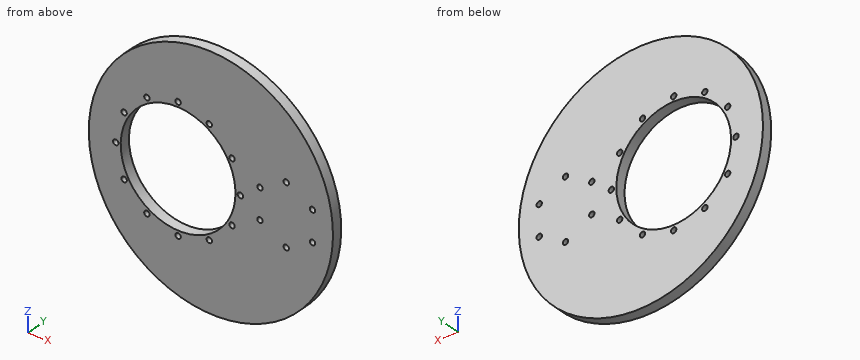
from build123d import *

# Parameters (mm, degrees)
SKETCH1_R                       = 74.45
SKETCH1_R_2                     = 35
BOSS_EXTRUDE1_DEPTH             = 6.35
M4X0_7_TAPPED_HOLE1_D           = 3.3
M4X0_7_TAPPED_HOLE1_ON_FACE_2_D = 3.3


with BuildPart() as part:
    # Sketch1 → Boss-Extrude1 (new body)
    with BuildSketch(Plane(origin=(0, 0, 0), x_dir=(1, 0, 0), z_dir=(0, 1, 0))):
        with Locations(Location((20, 0, 0), (0, 0, 270))):
            Circle(SKETCH1_R)
        with Locations(Location((0, 0, 0), (0, 0, 270))):
            Circle(SKETCH1_R_2, mode=Mode.SUBTRACT)
    extrude(amount=BOSS_EXTRUDE1_DEPTH)

    # M4x0.7 Tapped Hole1 (through all)
    with Locations(Plane(origin=(0, 0, -38), x_dir=(0, 0, -1), z_dir=(0, -1, 0))):
        with Locations((0, 0), (-5.091034656, -19), (-19, -32.908965344), (-38, -38), (-57, -32.908965344), (-70.908965344, -19), (-76, 0), (-70.908965344, 19), (-57, 32.908965344), (-38, 38), (-5.091034656, 19), (-19, 32.908965344)):
            Hole(M4X0_7_TAPPED_HOLE1_D / 2)

    # M4x0.7 Tapped Hole1 on face 2 (through all)
    with Locations(Plane(origin=(65.95, 6.35, -18.5), x_dir=(0, 0, 1), z_dir=(0, 1, 0))):
        with Locations((0, 0), (9.25, 16.02146997), (27.75, 16.02146997), (37, 0), (27.75, -16.02146997), (9.25, -16.02146997)):
            Hole(M4X0_7_TAPPED_HOLE1_ON_FACE_2_D / 2)


solid = part.part
Work out the finished part from the listing and answer in its coordinate system (mm). Round coordinates to 2 decimals unless told otherwise and drop trailing zeros. Loops run counter-clockwise (first coordinate to the right, second up) from the corner with the lowest first, then second, coordinate; pieces in that order, holes last. Notation, with made-up numbers: (73.25, 36.25) - (98.25, 36.25) arc R18 cw to (98.25, 68.25) - close; hole circle Ø8 at (8.5, 19.25). An arc over 180 degrees is marked (long way). Use one line per item in the form item = value. Start each with the question number.
(1) Find section A-A on x = -12. Determine the outline of the cut face in (y, z).
(2) Find section B-B on y = 4.25. Give the number of separate pieces and of enclosed holes in the cut face, and give its area (3 significant figures).
(3) Find section D-D on x = 69.5. Determine the outline of the cut face in (y, z), and give its area (3 significant figures).
(4) Flat-ended cylindrical pins translate along their axes: P1, Ø1.5, axis at x = 43.5, y = 1, coming from the -Z side; P2, Ø1.5, axis at y = 4, z = -50, coming from the -X side; P3, Ø3, axis at x = 25.5, y = 2, coming from the +Z side. Find the tip coordinate at first contact, or state that the pin passes through.
(5) Find section C-C on z = 42. Determine the outline of the cut face in (x, y).
(6) Consider line 1 (X direction, y = 3, z = 0); line 2 (Z direction, x = 51, y = 4); line 3 (Z direction, x = 67, y = 5). Determine where each line is inside the solid, lowest interval first.
Answer list:
q1.outline = (0, -67.22) - (6.35, -67.22) - (6.35, -32.88) - (0, -32.88) - close; (0, 32.88) - (6.35, 32.88) - (6.35, 67.22) - (0, 67.22) - close
q2.separate_pieces = 1
q2.enclosed_holes = 19
q2.area = 13,400 mm^2
q3.outline = (0, -55.61) - (6.35, -55.61) - (6.35, 55.61) - (0, 55.61) - close
q3.area = 706 mm^2
q4.P1 = -70.89
q4.P2 = -35.83
q4.P3 = 74.34
q5.outline = (-41.47, 0) - (81.47, 0) - (81.47, 6.35) - (-41.47, 6.35) - close
q6.line_1 = -54.45 to -39.65, -36.35 to -35, 35 to 36.35, 39.65 to 94.45
q6.line_2 = -67.69 to -10.5, -8 to 8, 10.5 to 67.69
q6.line_3 = -57.74 to -19.77, -17.23 to 17.23, 19.77 to 57.74
